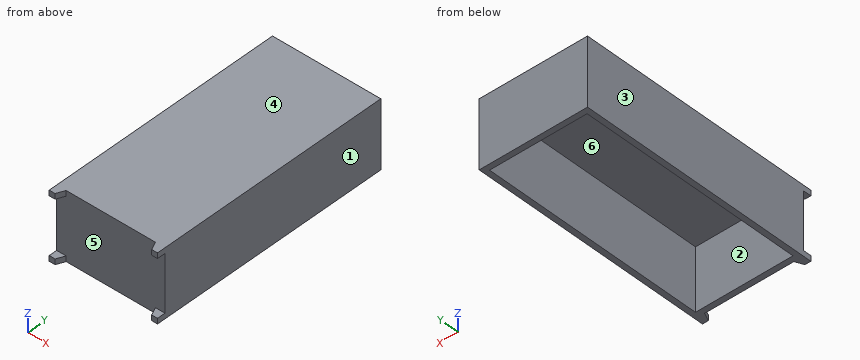
from build123d import *

# Parameters (mm, degrees)
BOSS_EXTRUDE1_DEPTH = 63.5
BOSS_EXTRUDE2_DEPTH = 5.08
BOSS_EXTRUDE3_START = 63.5
BOSS_EXTRUDE3_DEPTH = 5.08
SHELL1_OUTLINE_W    = 91.44
SHELL1_OUTLINE_H    = 210.82
SHELL1_DEPTH        = 58.42


# Read off the part's stored shape, not the designer's step: Shell1
with BuildPart() as part:
    # Sketch1 → Boss-Extrude1 (new body)
    with BuildSketch(Plane.XY):
        Polygon((-50.8, -106.68), (-41.900534076, -106.68), (41.900534076, -106.68), (50.8, -106.68), (50.8, 114.3), (-50.8, 114.3), align=None)
    extrude(amount=BOSS_EXTRUDE1_DEPTH)

    # Sketch1<4> → Boss-Extrude2 (add)
    with BuildSketch(Plane.XY):
        Polygon((50.8, -106.68), (41.900534076, -106.68), (45.287200742, -114.3), (50.8, -114.3), align=None)
        Polygon((-50.8, -114.3), (-45.287200742, -114.3), (-41.900534076, -106.68), (-50.8, -106.68), align=None)
    extrude(amount=BOSS_EXTRUDE2_DEPTH)

    # Sketch1<5> → Boss-Extrude3 (add)
    with BuildSketch(Plane.XY.offset(BOSS_EXTRUDE3_START)):
        Polygon((-50.8, -114.3), (-45.287200742, -114.3), (-41.900534076, -106.68), (-50.8, -106.68), align=None)
        Polygon((50.8, -106.68), (41.900534076, -106.68), (45.287200742, -114.3), (50.8, -114.3), align=None)
    extrude(amount=-BOSS_EXTRUDE3_DEPTH)

    # Shell1 outline → Shell1 (cut)
    with BuildSketch(Plane.XY):
        with Locations((0, 3.81)):
            Rectangle(SHELL1_OUTLINE_W, SHELL1_OUTLINE_H)
    extrude(amount=SHELL1_DEPTH, mode=Mode.SUBTRACT)


solid = part.part
Here's how the part is built. I have some questions about the finished solid (model axes, mm). Face numbers are marked on the shaded views. A direction names the side the tool comes from. Coordinates: 2 decimals unless noted, no trailing zeros. Order: outer loops, then holes, each group sorted by start corner. A loop starts at its lowest first (then second) coordinate and runs counter-clockwise, first axis right, second up.
Item 1: If we section it at B-B on x = -17.5: List the corners of the cut face in (y, z) for me, plus the area to 3 significant figures.
Result sheet:
outline: (-106.68, 0) - (-101.6, 0) - (-101.6, 58.42) - (109.22, 58.42) - (109.22, 0) - (114.3, 0) - (114.3, 63.5) - (-106.68, 63.5) - close
area: 1,720 mm2
Item 2: I need wall thicknesses on line 1 (X direction, y = 63.5, z = 52.5); line 2 (Y direction, x = 37.5, z = 14); line 3 (Y direction, x = -47, z = 10.5). Which ranges of each line are inside material? Lowest first, please.
Result sheet:
line 1: x = -50.8 to -45.72, 45.72 to 50.8
line 2: y = -106.68 to -101.6, 109.22 to 114.3
line 3: y = -106.68 to 114.3
Item 3: If we section it at A-A on z = 23.5: List the corners of the cut face in (x, y) for me.
Result sheet:
outline: (-50.8, -106.68) - (50.8, -106.68) - (50.8, 114.3) - (-50.8, 114.3) - close; hole (-45.72, -101.6) - (45.72, -101.6) - (45.72, 109.22) - (-45.72, 109.22) - close
Item 4: If we mould it in two halves opening along Z, with no side actions, what happens to the marked faces 3, 4, 5 and 6? For each: +Z half, -Z half, draft (parallel to the pull), parting line (faces both ways), or undercut.
Result sheet:
face 3: draft
face 4: +Z half
face 5: undercut
face 6: -Z half
Item 5: If we section it at C-C on y = 90: List the corners of the cut face in (x, z) for me, plus the area to 3 significant figures.
Result sheet:
outline: (-50.8, 0) - (-45.72, 0) - (-45.72, 58.42) - (45.72, 58.42) - (45.72, 0) - (50.8, 0) - (50.8, 63.5) - (-50.8, 63.5) - close
area: 1,110 mm2
Item 6: For P1, Ø4, axis at x = 12.5, y = -33.5, coming from the -Z side; P2, Ø12, axis at x = -9, z = 26, coming from the -Y side, each with a flat end and sliding along its axis, tell me the tip position at first contact or that it passes through.
Result sheet:
P1: stops at z = 58.42
P2: stops at y = -106.68
Item 7: For the marked faces 1 and 2, which set-ups out of +Z, -Z, +X, -X, +Y, -Y let a thin tool reach every point of the face, with its end or its side?
Result sheet:
face 1: +Z, -Z, +X, +Y, -Y
face 2: -Z
